Input: dimensioned drawing with shaded views. Units: mm. Origin: part minimum x, y, z. Round coordinates to 2 decimals unless told otherwise and drop trailing zeros. Write each loop counter-clockwise with the first axis right and the second up, starting at its lowest first coordinate (ties: lowest second). Pieces come first, ordered by that corner, then holes. Notation, with made-up numbers: M 30,36 L 68,36 A20 ccw 68,65 Z; hole C 38,79 d1. An arc over 180 degrees is marked long. Answer in a Markdown table with one row per item. Add a question column.
Item 1: Material intervals for probe 1 along Z at (x, y) = (31, 17); probe 2 along Y at (x, z) = (52, 4.3); probe 3 along Y at (x, z) = (57, 3.6) (1 decimal), sorted ascending.
Item 2: Cut plane C-C on y = 6.5. Return loops of the section in (x, z), and give its area (3 significant figures).
Item 3: Contact query for flat-ended pins moving along their axis: pin 1 (5 mm diameter, centred on x = 28.5, y = 36, fed in from +Z); pin 2 (1 mm diameter, centred on y = 44.5, z = 1.5, fed in from -X); pin 3 (3.5 mm diameter, centred on y = 66, z = 2.5, fed in from -X); pin 4 (5 mm diameter, centred on x = 8.5, y = 42.5, fed in from -Z). Output: stop coordinate, or through.
Item 4: Mould query, pull axis Y, two halves, no side actions, for the marked faces 1, 2 and 3. Classes: released by +Y, released by -Y, zero draft, split by the parting line, or undercut.
Item 5: Cut plane A-A on z = 3.4. Return loops of the section in (x, y), and give its area (3 significant figures).
Item 6: Cut plane D-D on x = 34. Return loops of the section in (y, z).
Item 7: Cut plane B-B on x = 42. Return loops of the section in (y, z), and give its area (3 significant figures).
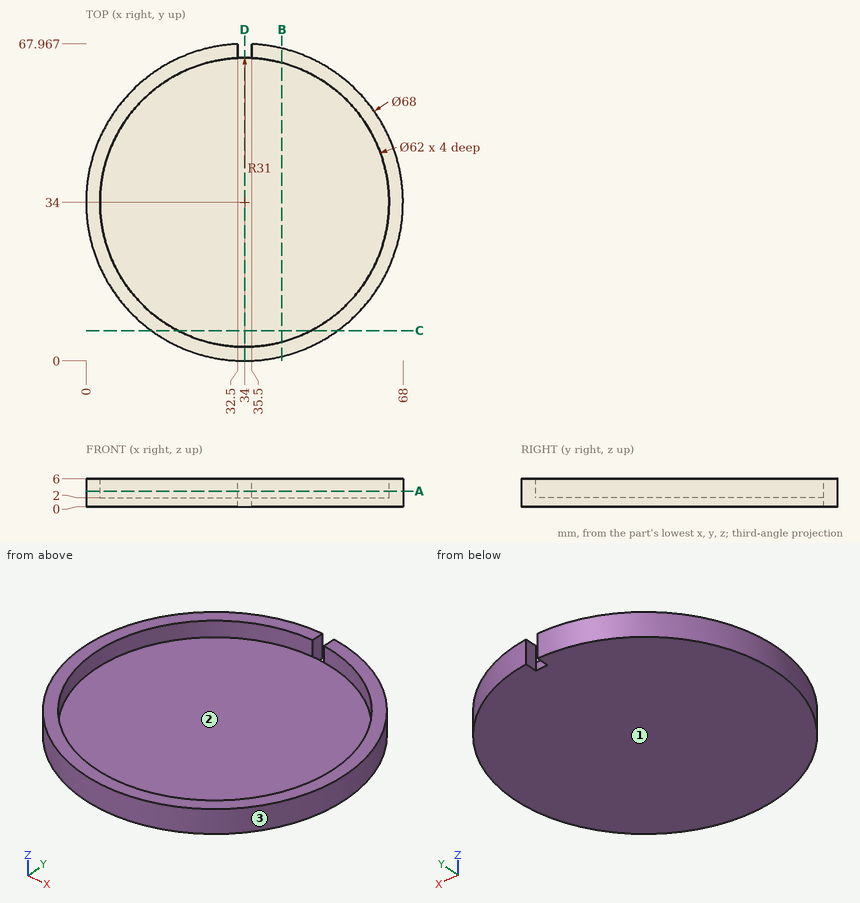
Results below:
| question | item | result |
|---|---|---|
| 1 | probe 1 | 0 to 2 |
| 1 | probe 2 | 5.16 to 8.76, 59.24 to 62.84 |
| 1 | probe 3 | 9 to 13.2, 54.8 to 59 |
| 2 | outline | M 14.01,0 L 53.99,0 L 53.99,6 L 48.31,6 L 48.31,2 L 19.69,2 L 19.69,6 L 14.01,6 Z |
| 2 | area | 125 mm2 |
| 3 | pin 1 | z = 2 |
| 3 | pin 2 | x = 1.5 |
| 3 | pin 3 | x = 18.48 |
| 3 | pin 4 | z = 0 |
| 4 | face 1 | zero draft |
| 4 | face 2 | undercut |
| 4 | face 3 | split by the parting line |
| 5 | outline | M 32.5,64.96 L 32.5,67.97 A34 ccw long 35.5,67.97 L 35.5,64.96 A31 cw long Z |
| 5 | area | 604 mm2 |
| 6 | outline | M 0,0 L 65,0 L 65,2 L 3,2 L 3,6 L 0,6 Z |
| 7 | outline | M 0.95,0 L 67.05,0 L 67.05,6 L 63.95,6 L 63.95,2 L 4.05,2 L 4.05,6 L 0.95,6 Z |
| 7 | area | 157 mm2 |
